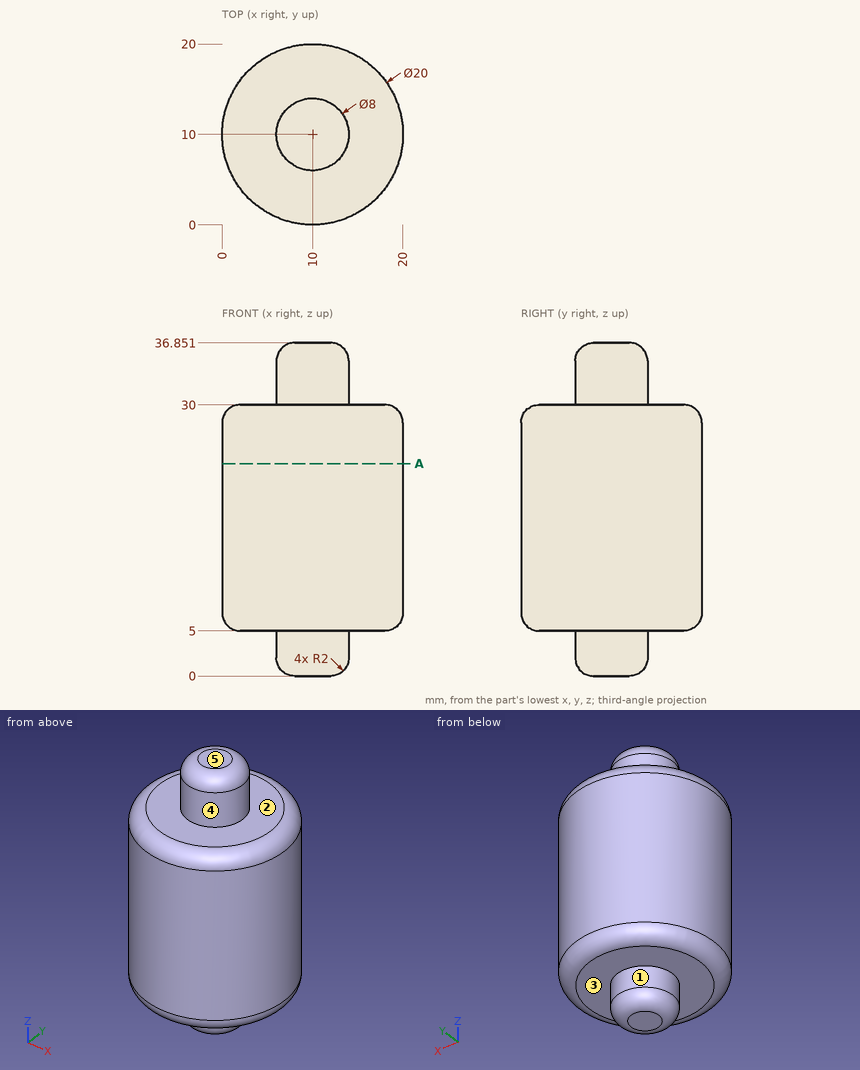
Print and shaded views of the part. All mm, measured from the part's lowest x, y and z. A direction names the side the tool comes from. Give positions to 0.01 mm unless a question says otherwise; leave off trailing zeros. Order: outer loops, then holes, each group sorted by start corner. A loop starts at its lowest first (then second) coordinate and runs counter-clockwise, first axis right, second up. Notation, with made-up numbers: (-24, 89.25) -> (28, 89.25) arc R15 cw to (28, 104.25) -> close; hole circle Ø1 at (-18.75, 39.25). An arc over 180 degrees is marked (long way). Use CSV: the item, a comma, the result in double quotes.
1. Mould opens along X. For the marked faces 1 and 2 say: +X half, -X half, draft (parallel to the pull), parting line (faces both ways), or undercut.
Outcome:
face 1,"parting line"
face 2,"draft"
2. Drill centre lines: line 1 along Z through (x, y) = (6.75, 12.5); line 2 along Y through (x, z) = (7, 18.5); line 3 along X through (y, z) = (16, 18). Where is each one in solid material? Low to high. Write a range as from..to.
Outcome:
line 1,"5..30"
line 2,"0.46..19.54"
line 3,"2..18"
3. Drop flat-ended pins along their axis: pin 1 (8 mm diameter, centred on y = 17.5, z = 8.5, fed in from +X); pin 2 (10 mm diameter, centred on x = 4.5, y = 2.5, fed in from +Z); pin 3 (5 mm diameter, centred on x = 5.5, z = 26.5, fed in from +Y). Give the stop position or say it passes through.
Outcome:
pin 1,"x = 19.37"
pin 2,"z = 30"
pin 3,"y = 19.8"
4. Band-saw the part on A-A, the plane z = 23.5. Give the cut face in (x, y), then the cut area to 3 significant figures.
Outcome:
outline,"circle Ø20 at (10, 10)"
area,"314 mm²"
5. 3-axis set-ups, long thin cutter, end or side, ignore diameter. For the marked faces 3, 4 and 5: which of +Z, -Z, +X, -X, +Y, -Y reach the whole face in a straight line?
Outcome:
face 3,"-Z"
face 4,"+Z"
face 5,"+Z, +X, -X, +Y, -Y"
